from build123d import *

# Parameters (mm, degrees)
F0_W     = 16
F0_H     = 16
F1_DEPTH = 8
F2_R     = 6
F3_DEPTH = 10


with BuildPart() as f1:
    # F0 (on Front) → F1 (new body, symmetric)
    with BuildSketch(Plane.XZ):
        Rectangle(F0_W, F0_H)
    extrude(amount=F1_DEPTH, both=True)

    # F2 (on Top) → F3 (join)
    with BuildSketch(Plane.XY):
        Circle(F2_R)
    extrude(amount=F3_DEPTH)


solid = f1.part
Geometry check sheet. Reference: the model listing, model coordinates, mm. A direction names the side the tool comes from. Give positions to 0.01 mm unless a question says otherwise; leave off trailing zeros. Write each loop counter-clockwise with the first axis right and the second up, starting at its lowest first coordinate (ties: lowest second). Pieces come first, ordered by that corner, then holes.
1) Cross-section at A-A (x = 0). Record the boundary of the cut face in (y, z).
Values follow:
outline: (-8, -8) - (8, -8) - (8, 8) - (6, 8) - (6, 10) - (-6, 10) - (-6, 8) - (-8, 8) - close
2) Cross-section at C-C (x = -6.5). Record the boundary of the cut face in (y, z), plus the area to 3 significant figures.
Values follow:
outline: (-8, -8) - (8, -8) - (8, 8) - (-8, 8) - close
area: 256 mm2
3) Thickness scan on line 1 (Z direction, x = -6.25, y = -2.75); line 2 (Y direction, x = 5.25, z = 8.25); line 3 (Y direction, x = -4, z = 9). Record the ranges inside material, lowest first.
Values follow:
line 1: z = -8 to 8
line 2: y = -2.9 to 2.9
line 3: y = -4.47 to 4.47
4) Set-up check for faces 1 (the face through (3.4, -5.4, 8)), 2 (the face through (0, 8, 0)): record each of +Z, -Z, +X, -X, +Y, -Y from which the full face is reachable in a straight line by a thin tool's end or side.
Values follow:
face 1: +Z
face 2: +Z, -Z, +X, -X, +Y
